Input: part model. Units: mm. Frame: model coordinates. Face numbers are marked on the shaded views. A direction names the side the tool comes from. Round coordinates to 2 decimals unless told otherwise and drop trailing zeros. Write each loop counter-clockwise with the first axis right and the second up, starting at its lowest first coordinate (ties: lowest second). Pieces come first, ordered by that corner, then holes. Notation, with made-up numbers: (32, 6) -> (80, 6) arc R18 ccw to (80, 29) -> close; hole circle Ø7 at (55, 4). An arc over 180 degrees is marked (long way). Write item = value, one per line.
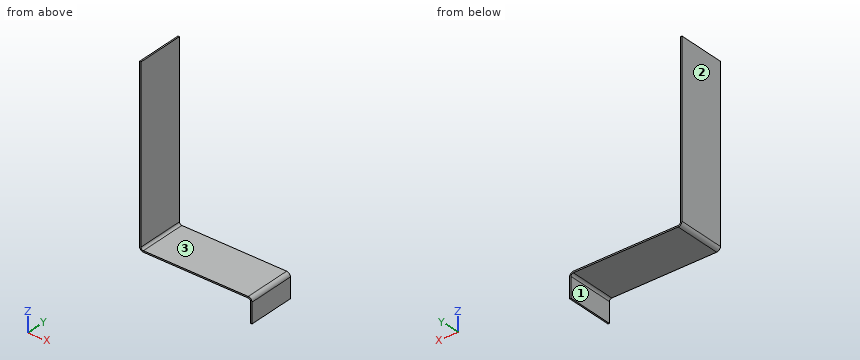
```python
from build123d import *

# Parameters (mm, degrees)
F1_DEPTH = 100


with BuildPart() as f1:
    # F0 (on Front) → F1 (new body)
    with BuildSketch(Plane.XZ):
        with BuildLine():
            ThreePointArc((0, -5), (-3.535534, -3.535534), (-5, 0))
            Line((-5, 0), (-5, 360))
            Line((-5, 360), (-8, 360))
            Line((-8, 360), (-8, 0))
            ThreePointArc((-8, 0), (-5.656854, -5.656854), (0, -8))
            Line((0, -8), (222, -8))
            ThreePointArc((222, -8), (225.535534, -9.464466), (227, -13))
            Line((227, -13), (227, -55.321693))
            Line((227, -55.321693), (230, -55.321693))
            Line((230, -55.321693), (230, -13))
            ThreePointArc((230, -13), (227.656854, -7.343146), (222, -5))
            Line((222, -5), (0, -5))
        make_face()
    extrude(amount=F1_DEPTH)


solid = f1.part
```
1) Cut plane A-A (y = -63). Return the cut outline in (x, z).
Solutions:
outline = (-8, 0) arc R8 ccw to (0, -8) -> (222, -8) arc R5 cw to (227, -13) -> (227, -55.32) -> (230, -55.32) -> (230, -13) arc R8 ccw to (222, -5) -> (0, -5) arc R5 cw to (-5, 0) -> (-5, 360) -> (-8, 360) -> close
2) Access query for the marked faces 1, 2 and 3. Directions: +Z, -Z, +X, -X, +Y, -Y. A direction counts if a zero-diameter tool reaches every point of the face in a straight line with its end or side. Return the directions, or none.
Solutions:
face_1 = -Z, -X, +Y, -Y
face_2 = +Z, -Z, -X, +Y, -Y
face_3 = +Z, +X, +Y, -Y
3) First-contact query: P1, Ø12, axis at y = -49.5, z = 204.5, coming from the +X side; P2, Ø1.5, axis at x = 146.5, y = -85, coming from the -Z side; P3, Ø12.5, axis at y = -61.5, z = -25.5, coming from the -X side. Flat tips, straight axial feed; report the tip coordinate or a pass-through.
Solutions:
P1 = -5
P2 = -8
P3 = 227
4) Cut plane C-C (z = 274). Return the cut outline in (x, y), and give its area (3 significant figures).
Solutions:
outline = (-8, -100) -> (-5, -100) -> (-5, 0) -> (-8, 0) -> close
area = 300 mm^2
5) Line query: L1, parallel to X at y = -87, z = 136.5; L2, parallel to X at y = -32, z = -31. Output: solid intervals per line, ascending. Write a range as from..to.
Solutions:
L1 = -8..-5
L2 = 227..230
6) Cut plane B-B (x = 195). Return the cut outline in (y, z).
Solutions:
outline = (-100, -8) -> (0, -8) -> (0, -5) -> (-100, -5) -> close
